The drawing under review shows one solid part. Ordinate dimensions are in mm from its lowest x, y, z. Coordinates: 2 decimals unless noted, no trailing zeros. Write each loop counter-clockwise with the first axis right and the second up, starting at its lowest first coordinate (ties: lowest second). Pieces come first, ordered by that corner, then holes.
Q1. Add section D-D, the plane x = 38.5. Give the boundary of the cut face in (y, z), plus the area to 3 significant figures.
Q2. Add section C-C, the plane y = 2.5. Give the number of separate pieces and of enclosed holes in the cut face, plus the area to 3 significant figures.
Q3. Add section A-A, the plane z = 45. Give the boundary of the cut face in (x, y).
Q4. To check wall thickness, follow probe 1 along X at (y, z) = (2.3, 45); probe 2 along Z at (x, y) = (55.5, 0.55); probe 3 along Z at (x, y) = (14, 1.3) (1 decimal). State the ranges of each line that lie inside material, in increasing order.
Q5. Clearance check with flat-ended pins moving along their axes: pin 1 Ø1.5 at (x, y) = (28, 1) entering from +Z; pin 2 Ø10 at (x, z) = (21.8, 20.2) entering from -Y; pin 3 Ø1.5 at (y, z) = (2, 21) entering from +X; pin 4 Ø1 at (y, z) = (1.5, 59) entering from -X. State where each tip first meets the part, or that it passes through.
Q6. Add section B-B, the plane x = 21.8. Give the boundary of the cut face in (y, z), plus the area to 3 significant figures.
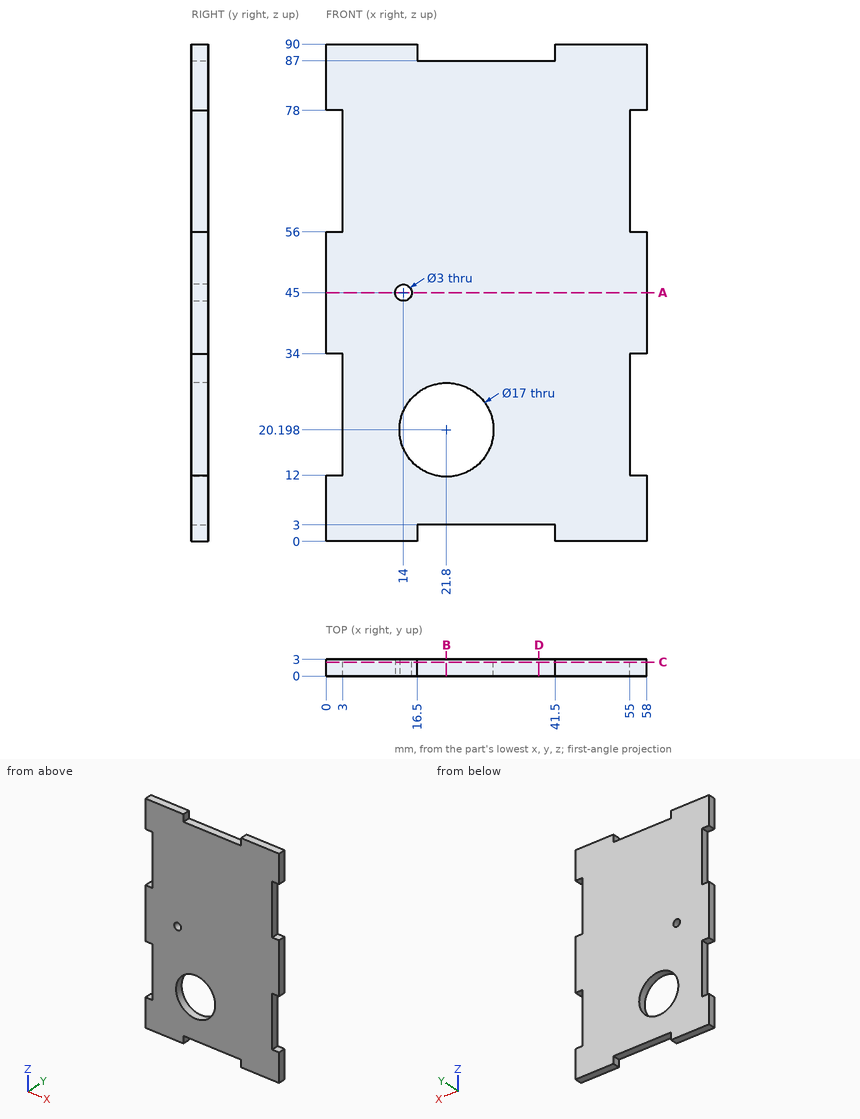
Here are the results:
1. outline: (0, 3) - (3, 3) - (3, 87) - (0, 87) - close
1. area: 252 mm2
2. separate pieces: 1
2. enclosed holes: 2
2. area: 4,570 mm2
3. outline: (0, 0) - (12.5, 0) - (12.5, 3) - (0, 3) - close; (15.5, 0) - (58, 0) - (58, 3) - (15.5, 3) - close
4. probe 1: x = 0 to 12.5, 15.5 to 58
4. probe 2: z = 0 to 12, 34 to 56, 78 to 90
4. probe 3: z = 0 to 16.8, 23.6 to 43.5, 46.5 to 90
5. pin 1: stops at z = 87
5. pin 2: passes through
5. pin 3: stops at x = 55
5. pin 4: stops at x = 3
6. outline: (0, 3) - (3, 3) - (3, 11.7) - (0, 11.7) - close; (0, 28.7) - (3, 28.7) - (3, 87) - (0, 87) - close
6. area: 201 mm2
